Here's how the part is built. I have some questions about the finished solid (model axes, mm). A direction names the side the tool comes from. Give positions to 0.01 mm unless a question says otherwise; leave off trailing zeros. Order: outer loops, then holes, each group sorted by start corner. A loop starts at its lowest first (then second) coordinate and runs counter-clockwise, first axis right, second up.
from build123d import *

# Parameters (mm, degrees)
F0_W     = 9.290261
F0_H     = 11.375831
F1_DEPTH = 25.4


with BuildPart() as f1:
    # F0 (on Right) → F1 (new body)
    with BuildSketch(Plane.YZ):
        Polygon((-35.454668, 24.647629), (-44.934526, 24.647629), (-44.934526, 9.859052), (-19.907702, 9.859052), (-19.907702, 24.647629), (-26.164407, 24.647629), align=None)
        with Locations((-30.809537, 30.335544)):
            Rectangle(F0_W, F0_H)
        Polygon((-9.479858, 9.859052), (-19.907702, 9.859052), (-19.907702, -2.65436), (-5.119123, -2.65436), (-5.119123, 5.498318), (-9.479858, 5.498318), align=None)
        with BuildLine():
            Line((-19.907702, 24.647629), (-19.907702, 9.859052))
            Line((-19.907702, 9.859052), (-9.479858, 9.859052))
            Line((-9.479858, 9.859052), (-5.119123, 9.859052))
            ThreePointArc((-5.119123, 9.859052), (-9.450598, 20.316156), (-19.907702, 24.647629))
        make_face()
    extrude(amount=F1_DEPTH)


solid = f1.part
Q1. For faces 5 (the face through (13, -35.455, 30)), 6 (the face through (13, -7, 5.498)), 7 (the face through (13, -23, 24.648)), which set-ups out of +Z, -Z, +X, -X, +Y, -Y let a thin tool reach every point of the face, with its end or its side?
Filled sheet:
face 5: +Z, +X, -X, -Y
face 6: +X, -X, +Y
face 7: +Z, +X, -X, +Y
Q2. Thinking about a two-plate mould opening in Z: for faces 1 (the face through (13, -31, 36.023)), 2 (the face through (13, -33, 9.859)), 3 (the face through (13, -7, 9.859)), 4 (the face through (25.4, -25, 17)), which applies, released by +Z, released by -Z, zero draft, split by the parting line, or undercut?
Filled sheet:
face 1: released by +Z
face 2: released by -Z
face 3: undercut
face 4: zero draft
Q3. If we section it at A-A on x = 14: List the corners of the cut face in (y, z) for me, plus the area to 3 significant figures.
Filled sheet:
outline: (-44.93, 9.86) - (-19.91, 9.86) - (-19.91, -2.65) - (-5.12, -2.65) - (-5.12, 5.5) - (-9.48, 5.5) - (-9.48, 9.86) - (-5.12, 9.86) arc R14.79 ccw to (-19.91, 24.65) - (-26.16, 24.65) - (-26.16, 36.02) - (-35.45, 36.02) - (-35.45, 24.65) - (-44.93, 24.65) - close
area: 814 mm2
Q4. I need wall thicknesses on L1, parallel to Z at x = 16, y = -22; L2, parallel to Y at x = 3, z = 0.5; L3, parallel to Z at x = 14.5, y = -27. Which ranges of each line are inside material? Lowest first, please.
Filled sheet:
L1: z = 9.86 to 24.65
L2: y = -19.91 to -5.12
L3: z = 9.86 to 36.02
Q5. If we section it at C-C on y = -25.5: List the corners of the cut face in (x, z) for me.
Filled sheet:
outline: (0, 9.86) - (25.4, 9.86) - (25.4, 24.65) - (0, 24.65) - close
Q6. If we section it at B-B on z = 4.5: List the corners of the cut face in (x, y) for me, plus the area to 3 significant figures.
Filled sheet:
outline: (0, -19.91) - (25.4, -19.91) - (25.4, -5.12) - (0, -5.12) - close
area: 376 mm2
Q7. I'm going to push flat-ended pins straight in: P1, Ø3.5, axis at x = 9.5, z = 8, coming from the +Y side; P2, Ø5, axis at y = -22.5, z = 23.5, coming from the -X side; P3, Ø1.5, axis at x = 6.5, z = 32, coming from the -Y side; P4, Ø12, axis at x = 3, y = -40.5, coming from the -Z side. Where does each tip first touch, or does it pass through?
Filled sheet:
P1: stops at y = -9.48
P2: stops at x = 0
P3: stops at y = -35.45
P4: stops at z = 9.86
